Source: CAD feature listing. Evaluate the final solid. Frame: model axes, mm. Give positions to 0.01 mm unless a question says otherwise; leave off trailing zeros. Write each loop counter-clockwise with the first axis right and the second up, starting at its lowest first coordinate (ties: lowest second). Pieces come first, ordered by that corner, then holes. Notation, with made-up numbers: M 25,68.5 L 41,68.5 A18 ccw 41,92.5 Z; hole C 2.25,62.5 d9. An arc over 180 degrees is marked long. Return JSON: item names as keys, results as strings.
```python
from build123d import *

# Parameters (mm, degrees)
CROQUIS1_W              = 8
CROQUIS1_H              = 6
SALIENTE_EXTRUIR1_DEPTH = 25
CROQUIS2_W              = 4
CROQUIS2_H              = 3
CORTAR_EXTRUIR1_DEPTH   = 27.019223663
CROQUIS3_R              = 1.5
CORTAR_EXTRUIR2_DEPTH   = 3
CROQUIS4_R              = 4
CROQUIS4_R_2            = 1.5
SALIENTE_EXTRUIR2_DEPTH = 3
CORTAR_EXTRUIR3_DEPTH   = 27.019223663
CORTAR_EXTRUIR4_DEPTH   = 3


with BuildPart() as part:
    # Croquis1 → Saliente-Extruir1 (new body)
    with BuildSketch(Plane.XY):
        Rectangle(CROQUIS1_W, CROQUIS1_H)
    extrude(amount=SALIENTE_EXTRUIR1_DEPTH)

    # Croquis2 → Cortar-Extruir1 (cut, through all)
    with BuildSketch(Plane(origin=(0, 3, 0), x_dir=(1, 0, 0), z_dir=(0, 1, 0))):
        with Locations((-2, -23.5)):
            Rectangle(CROQUIS2_W, CROQUIS2_H)
    extrude(amount=-CORTAR_EXTRUIR1_DEPTH, mode=Mode.SUBTRACT)

    # Croquis3 → Cortar-Extruir2 (cut)
    with BuildSketch(Plane.XZ.offset(3)):
        with Locations(Location((0, 7, 0), (0, 0, 270))):
            Circle(CROQUIS3_R)
    extrude(amount=-CORTAR_EXTRUIR2_DEPTH, mode=Mode.SUBTRACT)

    # Croquis4 → Saliente-Extruir2 (add)
    with BuildSketch(Plane.XZ.offset(3)):
        with Locations((0, 7)):
            Circle(CROQUIS4_R)
        with Locations(Location((0, 7, 0), (0, 0, 270))):
            Circle(CROQUIS4_R_2, mode=Mode.SUBTRACT)
    extrude(amount=-SALIENTE_EXTRUIR2_DEPTH)

    # Croquis5 → Cortar-Extruir3 (cut, through all)
    with BuildSketch(Plane(origin=(0, 3, 0), x_dir=(1, 0, 0), z_dir=(0, 1, 0))):
        with BuildLine():
            Line((4, 0), (-4, 0))
            Line((-4, 0), (-4, -7))
            ThreePointArc((-4, -7), (0, -3), (4, -7))
            Line((4, -7), (4, 0))
        make_face()
        with BuildLine():
            ThreePointArc((1.5, -7), (0, -5.5), (-1.5, -7))
            Line((-1.5, -7), (1.5, -7))
        make_face()
        with BuildLine():
            Line((1.5, -7), (-1.5, -7))
            ThreePointArc((-1.5, -7), (0, -8.5), (1.5, -7))
        make_face()
    extrude(amount=-CORTAR_EXTRUIR3_DEPTH, mode=Mode.SUBTRACT)

    # Croquis6 → Cortar-Extruir4 (cut)
    with BuildSketch(Plane.XY.offset(25)):
        with BuildLine():
            Line((0, 3), (0, 0))
            ThreePointArc((0, 0), (0.115822742, 1.517576993), (0.460607986, 3))
            Line((0.460607986, 3), (0, 3))
        make_face()
        with BuildLine():
            Line((0, 0), (0, -3))
            Line((0, -3), (0.460607986, -3))
            ThreePointArc((0.460607986, -3), (0.115822742, -1.517576993), (0, 0))
        make_face()
    extrude(amount=-CORTAR_EXTRUIR4_DEPTH, mode=Mode.SUBTRACT)


solid = part.part
```
1) Cut plane C-C, the plane z = 6.25. Return the cut outline in (x, y).
Numbers:
{"outline": "M -3.93,-3 L -1.3,-3 L -1.3,3 L -3.93,3 Z; M 1.3,-3 L 3.93,-3 L 3.93,3 L 1.3,3 Z"}
2) Contact query for flat-ended pins moving along their axis: pin 1 Ø1.8 at (x, z) = (0, 7) entering from +Y; pin 2 Ø1 at (y, z) = (-1, 5.5) entering from +X; pin 3 Ø3 at (x, y) = (-2, 0) entering from +Z. Output: stop coordinate, or through.
Numbers:
{"pin 1": "passes through", "pin 2": "stops at x = 3.87", "pin 3": "stops at z = 22"}
3) Cut plane B-B, the plane x = -0.75. Return the cut outline in (y, z), then the cut area to 3 significant figures.
Numbers:
{"outline": "M -3,3.07 L 3,3.07 L 3,5.7 L -3,5.7 Z; M -3,8.3 L 3,8.3 L 3,22 L -3,22 Z", "area": "98.0 mm²"}
4) Line query: line 1 (Z direction, x = 0, y = 2.35); line 2 (X direction, y = 1.2, z = 7); line 3 (Z direction, x = -1.25, y = -0.1). Output: solid intervals per line, ascending. Write a range as [from, to].
Numbers:
{"line 1": "z = [3, 5.5], [8.5, 22]", "line 2": "x = [-4, -1.5], [1.5, 4]", "line 3": "z = [3.2, 6.17], [7.83, 22]"}
5) Cut plane D-D, the plane y = 0.35. Return the cut outline in (x, z), then the cut area to 3 significant figures.
Numbers:
{"outline": "M -4,7 A4 ccw 4,7 L 4,25 L 0.01,25 L 0.01,22 L -4,22 Z; hole C 0,7 d3", "area": "150 mm²"}
6) Cut plane A-A, the plane y = 2.3. Return the cut outline in (x, z).
Numbers:
{"outline": "M -4,7 A4 ccw 4,7 L 4,25 L 0.27,25 L 0.27,22 L -4,22 Z; hole C 0,7 d3"}
